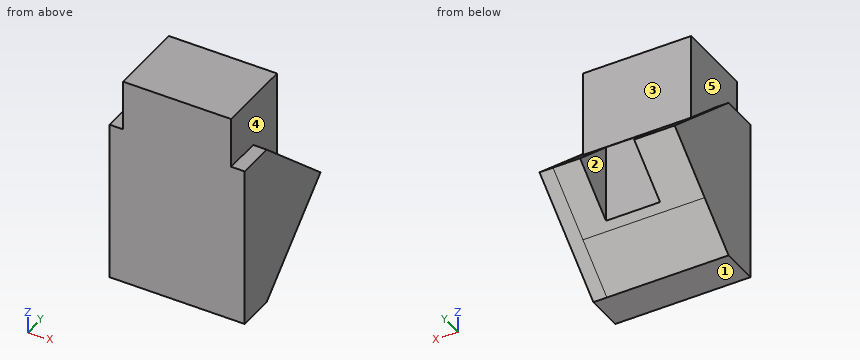
from build123d import *

# Parameters (mm, degrees)
CROQUIS1_W              = 40
CROQUIS1_H              = 63
SALIENTE_EXTRUIR1_DEPTH = 38
CROQUIS2_W              = 4
CROQUIS2_H              = 15
CORTAR_EXTRUIR1_DEPTH   = 38
CORTAR_EXTRUIR2_DEPTH   = 4
CORTAR_EXTRUIR14_DEPTH  = 60
CORTAR_EXTRUIR15_DEPTH  = 40
CROQUIS20_W             = 25.666666667
CROQUIS20_H             = 15
CROQUIS20_W_2           = 10.666666667
CORTAR_EXTRUIR16_DEPTH  = 40
CROQUIS22_W             = 16
CROQUIS22_H             = 13
CORTAR_EXTRUIR17_DEPTH  = 72
CORTAR_EXTRUIR19_DEPTH  = 40
SALIENTE_EXTRUIR2_DEPTH = 36
CORTAR_EXTRUIR20_DEPTH  = 4


with BuildPart() as part:
    # Croquis1 → Saliente-Extruir1 (new body)
    with BuildSketch(Plane(origin=(0, 0, 0), x_dir=(1, 0, 0), z_dir=(0, 1, 0))):
        with Locations((20, 31.5)):
            Rectangle(CROQUIS1_W, CROQUIS1_H)
    extrude(amount=SALIENTE_EXTRUIR1_DEPTH)

    # Croquis2 → Cortar-Extruir1 (cut)
    with BuildSketch(Plane(origin=(0, 38, 0), x_dir=(1, 0, 0), z_dir=(0, 1, 0))):
        with Locations((2, 7.5)):
            Rectangle(CROQUIS2_W, CROQUIS2_H)
        with Locations((38, 7.5)):
            Rectangle(CROQUIS2_W, CROQUIS2_H)
    extrude(amount=-CORTAR_EXTRUIR1_DEPTH, mode=Mode.SUBTRACT)

    # Croquis5 → Cortar-Extruir2 (cut)
    with BuildSketch(Plane(origin=(40, 0, 0), x_dir=(0, 0, -1), z_dir=(1, 0, 0))):
        Polygon((15, 38), (15, 11), (39, 38), align=None)
        Polygon((63, 38), (39, 38), (63, 11), align=None)
    extrude(amount=-CORTAR_EXTRUIR2_DEPTH, mode=Mode.SUBTRACT)

    # Croquis11 → Cortar-Extruir14 (cut)
    with BuildSketch(Plane(origin=(40, 0, 0), x_dir=(0, 0, -1), z_dir=(1, 0, 0))):
        Polygon((39, 38), (52.333333333, 23), (52.333333333, 38), align=None)
    extrude(amount=-CORTAR_EXTRUIR14_DEPTH, mode=Mode.SUBTRACT)

    # Croquis19 → Cortar-Extruir15 (cut)
    with BuildSketch(Plane(origin=(40, 0, 0), x_dir=(0, 0, -1), z_dir=(1, 0, 0))):
        Polygon((25.666666667, 23), (39, 38), (25.666666667, 38), align=None)
    extrude(amount=-CORTAR_EXTRUIR15_DEPTH, mode=Mode.SUBTRACT)

    # Croquis20 → Cortar-Extruir16 (cut)
    with BuildSketch(Plane(origin=(40, 0, 0), x_dir=(0, 0, -1), z_dir=(1, 0, 0))):
        with Locations((12.833333334, 30.5)):
            Rectangle(CROQUIS20_W, CROQUIS20_H)
        with Locations((57.666666667, 30.5)):
            Rectangle(CROQUIS20_W_2, CROQUIS20_H)
    extrude(amount=-CORTAR_EXTRUIR16_DEPTH, mode=Mode.SUBTRACT)

    # Croquis22 → Cortar-Extruir17 (cut)
    with BuildSketch(Plane.XY):
        with Locations((20, 31.5)):
            Rectangle(CROQUIS22_W, CROQUIS22_H)
    extrude(amount=-CORTAR_EXTRUIR17_DEPTH, mode=Mode.SUBTRACT)

    # Croquis23 → Cortar-Extruir19 (cut)
    with BuildSketch(Plane.ZY):
        Polygon((-63, 23), (-63, 11), (-52.333333333, 23), align=None)
        Polygon((-25.666666667, 23), (-15, 11), (-15, 23), align=None)
    extrude(amount=-CORTAR_EXTRUIR19_DEPTH, mode=Mode.SUBTRACT)

    # Croquis24 → Saliente-Extruir2 (add)
    with BuildSketch(Plane.ZY):
        Polygon((-15, 11), (-15, 23), (-25.666666667, 23), align=None)
    extrude(amount=-SALIENTE_EXTRUIR2_DEPTH)

    # Croquis26 → Cortar-Extruir20 (cut)
    with BuildSketch(Plane.ZY):
        Polygon((-15, 23), (-25.666666667, 23), (-15, 11), align=None)
    extrude(amount=-CORTAR_EXTRUIR20_DEPTH, mode=Mode.SUBTRACT)


solid = part.part
The listing builds one solid part. Answer for the finished solid, in the listing's coordinates (mm). Face numbers are marked on the shaded views. A direction names the side the tool comes from. Give positions to 0.01 mm unless a question says otherwise; leave off trailing zeros. Order: outer loops, then holes, each group sorted by start corner. A loop starts at its lowest first (then second) coordinate and runs counter-clockwise, first axis right, second up. Notation, with made-up numbers: (17.5, 27) - (59.5, 27) arc R23 ccw to (59.5, 64) - close; hole circle Ø2 at (86, 0). An arc over 180 degrees is marked (long way). Answer as CSV lines item,"result".
Q1. Which of the six approach directions +Z, -Z, +X, -X, +Y, -Y give full straight-line access (tool end or side, diameter ignored) to the marked faces 1, 2, 3, 4 and 5?
Answer key:
face 1,"-Z, +X, -X, +Y, -Y"
face 2,"+Z, -Z, +Y"
face 3,"+Z, +X, -X, +Y"
face 4,"+Z, +X, +Y"
face 5,"+Z, -X, +Y"
Q2. A cutting plane is placed at B-B, the plane x = 37. Determine the outline of the cut face in (y, z), and give its area (3 significant figures).
Answer key:
outline,"(0, -63) - (11, -63) - (38, -39) - (11, -15) - (0, -15) - close"
area,"1,180 mm^2"
Q3. A cutting plane is placed at A-A, the plane y = 6.5. Determine the outline of the cut face in (x, z).
Answer key:
outline,"(0, -63) - (40, -63) - (40, -15) - (36, -15) - (36, 0) - (4, 0) - (4, -15) - (0, -15) - close"
Q4. A cutting plane is placed at C-C, the plane z = -45. Determine the outline of the cut face in (x, y).
Answer key:
outline,"(0, 0) - (40, 0) - (40, 31.25) - (28, 31.25) - (28, 25) - (12, 25) - (12, 31.25) - (0, 31.25) - close"
Q5. Each of these flat-tipped pins is pushed along its axis until it touches: pin 1 Ø7.5 at (x, z) = (23.5, -8.5) entering from +Y; pin 2 Ø4 at (x, z) = (35, -42.5) entering from +Y; pin 3 Ø17.5 at (x, z) = (18, -44) entering from +Y; pin 4 Ø3 at (x, y) = (1, 5.5) entering from +Z. Where does it stop, or does it pass through?
Answer key:
pin 1,"stops at y = 23"
pin 2,"stops at y = 36.31"
pin 3,"stops at y = 38"
pin 4,"stops at z = -15"
Q6. A cutting plane is placed at D-D, the plane x = 31. Determine the outline of the cut face in (y, z), and give its area (4 significant figures).
Answer key:
outline,"(0, -63) - (11, -63) - (38, -39) - (23, -25.67) - (23, 0) - (0, 0) - close"
area,"1,585 mm^2"
Q7. Straight lines are drawn through the part: L1, parallel to X at y = 28, z = -45; L2, parallel to X at y = 6, z = -7; L3, parallel to Y at x = 20, z = -49. For each, find the intervals that lie inside material, in ascending order.
Answer key:
L1,"x = 0 to 12, 28 to 40"
L2,"x = 4 to 36"
L3,"y = 0 to 25"
